Part model, mm, in its own coordinate system. Round coordinates to 2 decimals unless told otherwise and drop trailing zeros. Loops run counter-clockwise (first coordinate to the right, second up) from the corner with the lowest first, then second, coordinate; pieces in that order, holes last.
from build123d import *

# Parameters (mm, degrees)
SKETCH1_W               = 203.2
SKETCH1_H               = 546.1
BOSS_EXTRUDE1_DEPTH     = 19.05
SKETCH2_R               = 19.2405
CUT_EXTRUDE1_DEPTH      = 583.990868282
ENL_V_MAT_EXTRU_1_REACH = 584.991
ESQUISSE1_R             = 15.875
ESQUISSE1_R_2           = 2.5


with BuildPart() as part:
    # Sketch1 → Boss-Extrude1 (new body)
    with BuildSketch(Plane.XY):
        with Locations((101.6, 273.05)):
            Rectangle(SKETCH1_W, SKETCH1_H)
    extrude(amount=BOSS_EXTRUDE1_DEPTH)

    # Sketch2 → Cut-Extrude1 (cut, through all)
    with BuildSketch(Plane(origin=(0, 0, 0), x_dir=(-1, 0, 0), z_dir=(0, 0, -1))):
        with Locations((-34.925, 495.3)):
            Circle(SKETCH2_R)
        with Locations((-34.925, 355.6)):
            Circle(SKETCH2_R)
    extrude(amount=-CUT_EXTRUDE1_DEPTH, mode=Mode.SUBTRACT)

    # Esquisse1 → Enlèv. mat.-Extru.1 (cut, up to next)
    with BuildSketch(Plane(origin=(0, 0, 0), x_dir=(-1, 0, 0), z_dir=(0, 0, -1)), mode=Mode.PRIVATE) as enl_v_mat_extru_1_sk1:
        with Locations((-34.925, 425.45)):
            Circle(ESQUISSE1_R)
    enl_v_mat_extru_1_tool1 = extrude(enl_v_mat_extru_1_sk1.sketch, amount=-ENL_V_MAT_EXTRU_1_REACH, mode=Mode.PRIVATE) & part.part
    # Esquisse1 → Enlèv. mat.-Extru.1 (cut, up to next)
    with BuildSketch(Plane(origin=(0, 0, 0), x_dir=(-1, 0, 0), z_dir=(0, 0, -1)), mode=Mode.PRIVATE) as enl_v_mat_extru_1_sk2:
        with Locations((-58.4962, 449.0212)):
            Circle(ESQUISSE1_R_2)
    enl_v_mat_extru_1_tool2 = extrude(enl_v_mat_extru_1_sk2.sketch, amount=-ENL_V_MAT_EXTRU_1_REACH, mode=Mode.PRIVATE) & part.part
    # Esquisse1 → Enlèv. mat.-Extru.1 (cut, up to next)
    with BuildSketch(Plane(origin=(0, 0, 0), x_dir=(-1, 0, 0), z_dir=(0, 0, -1)), mode=Mode.PRIVATE) as enl_v_mat_extru_1_sk3:
        with Locations((-11.3538, 449.0212)):
            Circle(ESQUISSE1_R_2)
    enl_v_mat_extru_1_tool3 = extrude(enl_v_mat_extru_1_sk3.sketch, amount=-ENL_V_MAT_EXTRU_1_REACH, mode=Mode.PRIVATE) & part.part
    # Esquisse1 → Enlèv. mat.-Extru.1 (cut, up to next)
    with BuildSketch(Plane(origin=(0, 0, 0), x_dir=(-1, 0, 0), z_dir=(0, 0, -1)), mode=Mode.PRIVATE) as enl_v_mat_extru_1_sk4:
        with Locations((-11.3538, 401.8788)):
            Circle(ESQUISSE1_R_2)
    enl_v_mat_extru_1_tool4 = extrude(enl_v_mat_extru_1_sk4.sketch, amount=-ENL_V_MAT_EXTRU_1_REACH, mode=Mode.PRIVATE) & part.part
    # Esquisse1 → Enlèv. mat.-Extru.1 (cut, up to next)
    with BuildSketch(Plane(origin=(0, 0, 0), x_dir=(-1, 0, 0), z_dir=(0, 0, -1)), mode=Mode.PRIVATE) as enl_v_mat_extru_1_sk5:
        with Locations((-58.4962, 401.8788)):
            Circle(ESQUISSE1_R_2)
    enl_v_mat_extru_1_tool5 = extrude(enl_v_mat_extru_1_sk5.sketch, amount=-ENL_V_MAT_EXTRU_1_REACH, mode=Mode.PRIVATE) & part.part
    add(enl_v_mat_extru_1_tool1.solids().sort_by_distance((34.925, 425.45, 0))[0], mode=Mode.SUBTRACT)
    add(enl_v_mat_extru_1_tool2.solids().sort_by_distance((58.4962, 449.0212, 0))[0], mode=Mode.SUBTRACT)
    add(enl_v_mat_extru_1_tool3.solids().sort_by_distance((11.3538, 449.0212, 0))[0], mode=Mode.SUBTRACT)
    add(enl_v_mat_extru_1_tool4.solids().sort_by_distance((11.3538, 401.8788, 0))[0], mode=Mode.SUBTRACT)
    add(enl_v_mat_extru_1_tool5.solids().sort_by_distance((58.4962, 401.8788, 0))[0], mode=Mode.SUBTRACT)


solid = part.part
1) Slice it at A-A, the plane y = 355.6. Give the cut face in (x, z), then the cut area to 3 significant figures.
Values:
outline: (0, 0) - (15.68, 0) - (15.68, 19.05) - (0, 19.05) - close; (54.17, 0) - (203.2, 0) - (203.2, 19.05) - (54.17, 19.05) - close
area: 3,140 mm2
2) Wall check: line 1 along Y through (x, z) = (52, 17); line 2 along Y through (x, z) = (31.5, 6.75); line 3 along Y through (x, z) = (23.5, 2.25). Give the ranges that are in metal, low to high.
Values:
line 1: y = 0 to 346.73, 364.47 to 486.43, 504.17 to 546.1
line 2: y = 0 to 336.67, 374.53 to 409.95, 440.95 to 476.37, 514.23 to 546.1
line 3: y = 0 to 340.12, 371.08 to 414.43, 436.47 to 479.82, 510.78 to 546.1
3) Slice it at B-B, the plane x = 36.5. Give the cut face in (y, z).
Values:
outline: (0, 0) - (336.42, 0) - (336.42, 19.05) - (0, 19.05) - close; (374.78, 0) - (409.65, 0) - (409.65, 19.05) - (374.78, 19.05) - close; (441.25, 0) - (476.12, 0) - (476.12, 19.05) - (441.25, 19.05) - close; (514.48, 0) - (546.1, 0) - (546.1, 19.05) - (514.48, 19.05) - close
4) Mould opens along X. For faces 1 (the face through (39.096, 336.817, 9.392)), 2 (the face through (36.99, 441.19, 9.39)), 3 (the face through (100, 277, 19.05)), 4 (the face through (203.2, 269, 9)) say: released by +X, released by -X, zero draft, split by the parting line, or undercut.
Values:
face 1: undercut
face 2: undercut
face 3: zero draft
face 4: released by +X
5) Slice it at C-C, the plane z = 16. Give the number of separate pieces and of enclosed holes in the cut face, then the cut area to 3 significant figures.
Values:
separate pieces: 1
enclosed holes: 7
area: 108,000 mm2
6) Slice it at D-D, the plane y = 425.45. Give the cut face in (x, z).
Values:
outline: (0, 0) - (19.05, 0) - (19.05, 19.05) - (0, 19.05) - close; (50.8, 0) - (203.2, 0) - (203.2, 19.05) - (50.8, 19.05) - close
